```python
from build123d import *

# Parameters (mm, degrees)
SKETCH1_R           = 19.05
SKETCH1_R_2         = 13.49375
BOSS_EXTRUDE1_DEPTH = 31.75
SKETCH2_R           = 15.875
CUT_EXTRUDE1_DEPTH  = 26.9875
CHAMFER1_SIZE       = 0.79375


with BuildPart() as part:
    # Sketch1 → Boss-Extrude1 (new body)
    with BuildSketch(Plane.XY):
        Circle(SKETCH1_R)
        Circle(SKETCH1_R_2, mode=Mode.SUBTRACT)
    extrude(amount=BOSS_EXTRUDE1_DEPTH)

    # Sketch2 → Cut-Extrude1 (cut)
    with BuildSketch(Plane.XY.offset(31.75)):
        Circle(SKETCH2_R)
    extrude(amount=-CUT_EXTRUDE1_DEPTH, mode=Mode.SUBTRACT)

    # Mirror1: part across plane


with BuildPart() as part_1:
    add(part.part)
    add(part.part.mirror(Plane.XY))

    # Chamfer1
    chamfer1_edges = [part_1.edges().sort_by_distance(p)[0] for p in [
        (-15.875, 0, 31.75),
        (-15.875, 0, -31.75),
    ]]
    chamfer(chamfer1_edges, length=CHAMFER1_SIZE)


solid = part_1.part
```
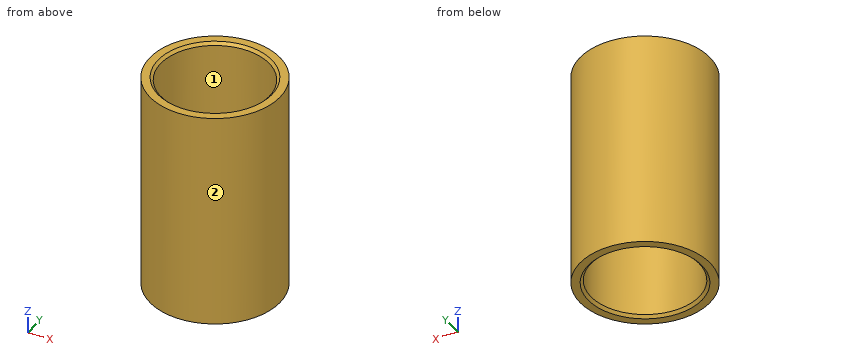
For this review, take the finished solid that the model builds, in its own axes (mm). Face numbers are marked on the shaded views. Give positions to 0.01 mm unless a question says otherwise; leave off trailing zeros. Write each loop counter-clockwise with the first axis right and the second up, starting at its lowest first coordinate (ties: lowest second). Pieces come first, ordered by that corner, then holes. Notation, with made-up numbers: M 54.25,41 L 97.25,41 A11 cw 97.25,54 Z; hole C 68.25,33 d11. An arc over 180 degrees is marked long. Answer as a JSON object with one key per item and string values. Group by question number.
Item 1: For probe 1 along Y at (x, z) = (0, -0.5); probe 2 along Z at (x, y) = (10.5, 9.5); probe 3 along Y at (x, z) = (-7, -4.5), list the stretches that pass through material, from the lowest coordinate up. Write a range as [from, to].
Item 2: Draft analysis for pull direction X (two halves, no side actions). For the marked faces 1 and 2, state which applies: +X half, -X half, draft (parallel to the pull), parting line (faces both ways), or undercut.
Item 3: Consider section C-C on z = -19. Write out the cut boundary in (x, y) (3 decimals).
Item 4: For pin 1 Ø4 at (y, z) = (2.5, -24.5) entering from +X; pin 2 Ø1 at (y, z) = (14.5, -19.5) entering from -X; pin 3 Ø9.5 at (x, y) = (7, -6.5) entering from -Z; pin 4 Ø16 at (x, y) = (0, 0) entering from +Z, all flat-tipped, find the tip position at first contact; note any pin that passes through.
Check result:
{
 "1": {"probe 1": "y = [-19.05, -13.49], [13.49, 19.05]", "probe 2": "z = [-4.76, 4.76]", "probe 3": "y = [-17.72, -11.54], [11.54, 17.72]"},
 "2": {"face 1": "undercut", "face 2": "parting line"},
 "3": {"outline": "C 0,0 d38.1; hole C 0,0 d31.75"},
 "4": {"pin 1": "stops at x = 19.04", "pin 2": "stops at x = -12.92", "pin 3": "stops at z = -4.76", "pin 4": "passes through"}
}
